Autodesk Inventor part; units mm, degrees
ref_plane "YZ Plane" through (0, 0, 0) normal (1, 0, 0) x (0, 1, 0)
ref_plane "XZ Plane" through (0, 0, 0) normal (0, 1, 0) x (-1, 0, 0)
ref_plane "XY Plane" through (0, 0, 0) normal (0, 0, 1) x (1, 0, 0)
sketch "Sketch1" plane through (0, 0, 0) normal (0, 1, 0) x (-1, 0, 0)
  circle A0 centre (0, 0) radius 62.05
  circle A1 centre (0, 0) radius 76
  dimension "d0" = 124.1
extrude "Extrusion1" add sketch "Sketch1" along normal blind 10
sketch "Sketch2" plane through (0, 10, 0) normal (0, 1, 0) x (1, 0, 0)
  circle A0 centre (0, 0) radius 76
  circle A1 centre (0, 0) radius 62.05
  line L0 (-76, 0) -> (76, 0)
  line L1 (76, 0) -> (76, 220)
  line L2 (76, 220) -> (-76, 220)
  line L3 (-76, 220) -> (-76, 0)
  line L4 (-126, 220) -> (126, 220)
  line L5 (126, 220) -> (126, 187)
  line L6 (126, 187) -> (-126, 187)
  line L7 (-126, 187) -> (-126, 220)
  line L8 (126, 187) -> (73.6534, -18.7397)
  circle A2 centre (0, 0) radius 76
  line L9 (-126, 187) -> (-73.6534, -18.7397)
  point P0 (-73.6534, -18.7397)
  point P1 (73.6534, -18.7397)
  dimension "d3" = 220
  dimension "d4" = 50
  dimension "d5" = 50
  dimension "d15" = 33
  dimension "d16" = 76
  dimension "d17" = 76
  dimension "d18" = 126
extrude "Extrusion2" add sketch "Sketch2" along normal blind 70
sketch "Sketch3" plane through (126, 10, -187) normal (1, 0, 0) x (0, 0, -1)
  line L0 (39, 50) -> (0, 50)
  line L1 (0, 0) -> (0, 70)
  line L2 (0, 50) -> (-111, 0)
  line L3 (-205.7397, 0) -> (0, 0)
  line L4 (39, 50) -> (39, 0)
  line L5 (39, 0) -> (-111, 0)
  line L6 (0, 70) -> (33, 70)
  point P0 (-187, -10)
  dimension "d10" = 20
extrude "Extrusion3" cut sketch "Sketch3" against normal blind 300
sketch "Sketch4" plane through (0, 10, 0) normal (0, -1, 0) x (1, 0, 0)
  circle A0 centre (0, 0) radius 58
  line L0 (-97.7581, -76) -> (97.7581, -76)
  circle A1 centre (0, 0) radius 76
  line L1 (126, -220) -> (-126, -220)
  line L2 (126, -187) -> (126, -220)
  line L3 (126, -187) -> (-126, -187)
  line L4 (-126, -220) -> (-126, -187)
  line L5 (97.7581, -76) -> (126, -187)
  line L6 (0, -76) -> (97.7581, -76)
  line L7 (-97.7581, -76) -> (0, -76)
  line L8 (-126, -187) -> (-97.7581, -76)
  line L9 (126, -187) -> (-126, -187)
  line L10 (0, -76) -> (97.7581, -76)
  line L11 (73.6534, 18.7397) -> (97.7581, -76)
  arc A2 (0, -76) -> (73.6534, 18.7397) centre (0, 0) ccw
  line L12 (-97.7581, -76) -> (0, -76)
  arc A3 (-73.6534, 18.7397) -> (0, -76) centre (0, 0) ccw
  line L13 (-97.7581, -76) -> (-73.6534, 18.7397)
  line L14 (64.6258, -26.8898) -> (109.6331, -203.7836)
  line L15 (-65.3309, -29.6614) -> (-109.9518, -205.0363)
  line L16 (8, -74) -> (-8, -74)
  line L17 (-8, -74) -> (-8, -228)
  line L18 (-8, -228) -> (8, -228)
  line L19 (8, -228) -> (8, -74)
  line L20 (0, -76) -> (97.7581, -76)
  circle A4 centre (0, 0) radius 62.05
  line L21 (73.6534, 18.7397) -> (97.7581, -76)
  arc A5 (0, -76) -> (73.6534, 18.7397) centre (0, 0) ccw
  line L22 (-97.7581, -76) -> (0, -76)
  circle A6 centre (0, 0) radius 62.05
  arc A7 (-73.6534, 18.7397) -> (0, -76) centre (0, 0) ccw
  line L23 (-97.7581, -76) -> (-73.6534, 18.7397)
  point P0 (-8, -75.5778)
  point P1 (-66.9402, -35.9863)
  point P2 (-105.3628, -187)
  point P3 (-8, -187)
  point P4 (8, -187)
  point P5 (105.3628, -187)
  point P6 (66.9402, -35.9863)
  point P7 (8, -75.5778)
  dimension "d11" = 20
  dimension "d12" = 20
extrude "Extrusion5" cut sketch "Sketch4" against normal blind 300 contours A0 | L15 A1 L17 L0 | L0 L17 L3 L15 | L19 A1 L14 L0 | L0 L14 L3 L19
chamfer "Chamfer1" distance 33 angle 45 6 edges at (-126, 70, -220) (126, 70, -220) (105.3628, 70, -187) (-105.3628, 70, -187) (8, 70, -187) (-8, 70, -187)
sketch "Sketch7" plane through (93, 60, -220) normal (0, 0, -1) x (-1, 0, 0)
  line L0 (0, 20) -> (186, 20)
  line L1 (0, 0) -> (186, 0)
  line L2 (125.5, 20) -> (60.5, 20)
  line L3 (60.5, 20) -> (60.5, 0)
  line L4 (60.5, 0) -> (125.5, 0)
  line L5 (125.5, 0) -> (125.5, 20)
  line L6 (186, 20) -> (186, 0)
  line L7 (0, 0) -> (0, 20)
  point P0 (93, -60)
  point P1 (125.5, 0)
  point P2 (60.5, 20)
  dimension "d24" = 65
  dimension "d25" = 60.5
  dimension "d26" = 60.5
extrude "Extrusion6" cut sketch "Sketch7" against normal blind 4 contours L0 L5 L1 L3
properties part number "KrovatkaShatunPods" material "Aluminum 6061-AHC"
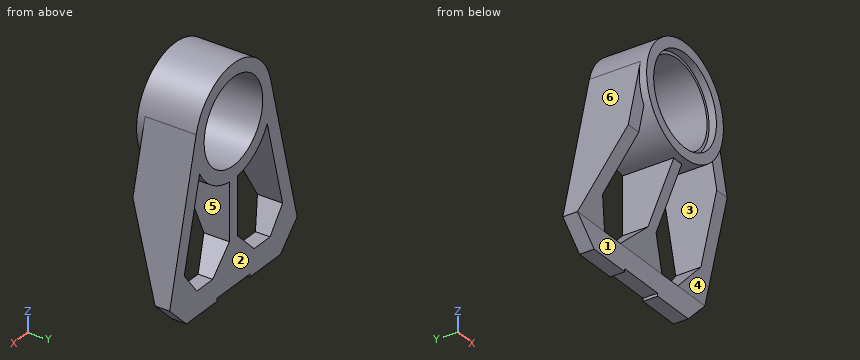
Build history of the part. All positions in model axes, mm. Face numbers are marked on the shaded views. A direction names the side the tool comes from. Round coordinates to 2 decimals unless told otherwise and drop trailing zeros. Order: outer loops, then holes, each group sorted by start corner. A loop starts at its lowest first (then second) coordinate and runs counter-clockwise, first axis right, second up. Notation, with made-up numbers: M 43,-15.5 L 93,-15.5 A16 ccw 93,-0.5 Z; hole C 63,-0.5 d4. An arc over 180 degrees is marked long. Use CSV: the item, a comma, the result in double quotes. Start each with the question number.
(1) Cut at B-B on y = 17.5. List the corners of the cut face in (x, z).
(2) Tool access for the marked faces 1, 2 and 3: list every direction of +Z, -Z, +X, -X, +Y, -Y with a clear straight run to the whole face (end or side of a thin tool).
(3) Drill centre lines: probe 1 along Z at (x, y) = (0, 4.5); probe 2 along Z at (x, y) = (0, 63.5); probe 3 along Z at (x, y) = (-21.5, 55). Where is each one in solid material? Low to high.
(4) Cut at C-C on x = 87. List the corners of the cut face in (y, z), then the cut area to 3 significant figures.
(5) Cut at D-D on z = -122.5. List the corners of the cut face in (x, y).
(6) Cut at A-A on z = 0. List the corners of the cut face in (x, y).
(7) Flat gauge pins, fed straight in: P1, Ø21, axis at y = 58, z = -116, coming from the +X side; P2, Ø3, axis at y = 44, z = 21.5, coming from the -X side; P3, Ø1.2, axis at y = 73, z = -217, coming from the -X side; P4, Ø1.5, axis at y = 24, z = -113.5, coming from the -X side. Where does each tip first touch, or does it go through?
(8) Mould opens along X. For the marked faces 4, 5 and 6 say: +X half, -X half, draft (parallel to the pull), parting line (faces both ways), or undercut.
Findings:
1,outline,"M -101.99,-92.65 L -81.36,-92.65 L -66.94,-35.99 A76 ccw -8,-75.58 L -8,-92.65 L 8,-92.65 L 8,-75.58 A76 ccw 66.94,-35.99 L 81.36,-92.65 L 101.99,-92.65 L 73.65,18.74 A76 ccw -73.65,18.74 Z; hole C 0,0 d116"
2,face 1,"-Z, +X, -X, -Y"
2,face 2,"+Z, -Z, +X, -X, +Y"
2,face 3,"+Y, -Y"
3,probe 1,"z = -76 to -62.05, 62.05 to 76"
3,probe 2,"z = -216 to -58, 58 to 76"
3,probe 3,"z = -175.9 to -167.5, -72.9 to -53.87, 53.87 to 72.9"
4,outline,"M 10,-76 L 27.49,-114.83 L 80,-114.83 L 80,-33.72 L 10,-33.72 Z; M 51.52,-168.17 L 60,-187 L 60,-220 L 80,-220 L 80,-168.17 Z"
4,area,"6,450 mm^2"
5,outline,"M -109.59,30.95 L -88.95,30.95 L -88.95,80 L -109.59,80 Z; M -8,30.95 L 8,30.95 L 8,80 L -8,80 Z; M 88.95,30.95 L 109.59,30.95 L 109.59,80 L 88.95,80 Z"
6,outline,"M -78.42,10 L -76,10 L -76,0 L -62.05,0 L -62.05,10 L -58,10 L -58,80 L -78.42,80 Z; M 58,10 L 62.05,10 L 62.05,0 L 76,0 L 76,10 L 78.42,10 L 78.42,80 L 58,80 Z"
7,P1,"stops at x = 110.61"
7,P2,"stops at x = -73.32"
7,P3,"stops at x = -96.6"
7,P4,"passes through"
8,face 4,"draft"
8,face 5,"undercut"
8,face 6,"-X half"
